```python
from build123d import *

# Parameters (mm, degrees)
F0_W     = 24.05
F0_H     = 19.09
F1_DEPTH = 9.02
F2_R     = 2
F4_DEPTH = 3.05
F5_W     = 11.32
F5_H     = 1.87
F6_DEPTH = 12.33


with BuildPart() as f1:
    # F0 (on Top) → F1 (new body)
    with BuildSketch(Plane.XY):
        Rectangle(F0_W, F0_H)
    extrude(amount=F1_DEPTH)

    # F2
    f2_edges = [f1.edges().sort_by_distance(p)[0] for p in [
        (12.025, -9.545, 4.51),
        (12.025, 9.545, 4.51),
        (-12.025, 9.545, 4.51),
        (-12.025, -9.545, 4.51),
    ]]
    fillet(f2_edges, radius=F2_R)

    # F3 (on face) → F4 (join)
    with BuildSketch(Plane.YZ.offset(12.025)):
        Polygon((0, 7.49), (-5.66, 7.49), (-5.66, 5.57), (5.66, 5.57), (5.66, 7.49), align=None)
    extrude(amount=F4_DEPTH)

    # F5 (on face) → F6 (join)
    with BuildSketch(Plane.YZ.offset(12.025)):
        with Locations((0, 4.635)):
            Rectangle(F5_W, F5_H)
    extrude(amount=F6_DEPTH)


solid = f1.part
```
Check sheet for the modelled part. Datum: model origin and axes. Units: mm. A direction names the side the tool comes from. Round coordinates to 2 decimals unless told otherwise and drop trailing zeros. Write each loop counter-clockwise with the first axis right and the second up, starting at its lowest first coordinate (ties: lowest second). Pieces come first, ordered by that corner, then holes. Notation, with made-up numbers: (-13.75, -3.75) -> (5.25, -3.75) arc R20 cw to (5.25, 32.25) -> close; hole circle Ø5 at (-9, 67). An arc over 180 degrees is marked (long way). One line per question, with ' | ' between items. Start each with the question number.
1. Sectioned sample at C-C, the plane x = 14.5. Record the cut outline in (y, z).
2. Scan lines: line 1 along X through (y, z) = (-7.25, 4.5) (3 decimals); line 2 along X through (y, z) = (4, 6) (3 decimals); line 3 along Y through (x, z) = (19, 5.5). Record each from-to range of solid material in increasing order. Write a range as from..to.
3. Sectioned sample at A-A, the plane y = 1.75. Record the cut outline in (x, z) (3 decimals).
4. Sectioned sample at D-D, the plane z = 8. Record the cut outline in (x, y) (3 decimals), then the cut area to 3 significant figures.
5. Set-up check for faces 1 (the face through (15.075, 0, 7)), 2 (the face through (17, 5.66, 5)), 3 (the face through (17, -5.66, 5)): record each of +Z, -Z, +X, -X, +Y, -Y from which the full face is reachable in a straight line by a thin tool's end or side.
6. Sectioned sample at B-B, the plane z = 6.5. Record the cut outline in (x, y) (3 decimals).
7. Depth check by flat-ended pin: pin 1 (10 mm diameter, centred on x = 21.5, y = -1, fed in from +Z); pin 2 (1 mm diameter, centred on x = 16, z = 2.5, fed in from -Y); pin 3 (1 mm diameter, centred on x = 13.5, y = -5.5, fed in from -Z); pin 4 (3 mm diameter, centred on x = 18, z = 6.5, fed in from +Y). Enter the tip coordinate at first touch or a pass-through.
Taken from the geometry:
1) outline: (-5.66, 3.7) -> (5.66, 3.7) -> (5.66, 7.49) -> (-5.66, 7.49) -> close
2) line 1: x = -12.025..12.025 | line 2: x = -12.025..15.075 | line 3: y = -5.66..5.66
3) outline: (-12.025, 0) -> (12.025, 0) -> (12.025, 3.7) -> (24.355, 3.7) -> (24.355, 5.57) -> (15.075, 5.57) -> (15.075, 7.49) -> (12.025, 7.49) -> (12.025, 9.02) -> (-12.025, 9.02) -> close
4) outline: (-12.025, -7.545) arc R2 ccw to (-10.025, -9.545) -> (10.025, -9.545) arc R2 ccw to (12.025, -7.545) -> (12.025, 7.545) arc R2 ccw to (10.025, 9.545) -> (-10.025, 9.545) arc R2 ccw to (-12.025, 7.545) -> close | area: 456 mm^2
5) face 1: +Z, +X, +Y, -Y | face 2: +Z, -Z, +X, +Y | face 3: +Z, -Z, +X, -Y
6) outline: (-12.025, -7.545) arc R2 ccw to (-10.025, -9.545) -> (10.025, -9.545) arc R2 ccw to (12.025, -7.545) -> (12.025, -5.66) -> (15.075, -5.66) -> (15.075, 5.66) -> (12.025, 5.66) -> (12.025, 7.545) arc R2 ccw to (10.025, 9.545) -> (-10.025, 9.545) arc R2 ccw to (-12.025, 7.545) -> close
7) pin 1: stops at z = 5.57 | pin 2: passes through | pin 3: stops at z = 3.7 | pin 4: stops at y = 5.66
